Verification items for this drawing (mm, ordinates from the low corner). A direction names the side the tool comes from. Give positions to 0.01 mm unless a question says otherwise; leave off trailing zeros. Loops run counter-clockwise (first coordinate to the right, second up) from the corner with the lowest first, then second, coordinate; pieces in that order, holes last. Notation, with made-up numbers: (43, 27.25) -> (52, 27.25) arc R17 cw to (52, 44.25) -> close; hole circle Ø2 at (55, 51.5). An arc over 180 degrees is marked (long way). Answer in a Markdown table with one row per item. Add a question column.
Q1. Material ranges on probe 1 along Y at (x, z) = (5, 6); probe 2 along Y at (x, z) = (17, 8.5); probe 3 along Y at (x, z) = (16, 2.5), recorded low to high.
Q2. Section check C-C on y = 16. Enter the section's corners in (x, z).
Q3. Section check D-D on y = 7. Enter the section's corners in (x, z).
Q4. Release check for a two-part mould opening along Y. For the marked faces 1, 2, 3 and 4 record: pulls with the +Y half, pulls with the -Y half, needs draft (parallel to the pull), parting line crosses it, or undercut.
Q5. Section check A-A on x = 5. Enter the section's corners in (y, z), and give its area (3 significant figures).
Q6. Section check B-B on z = 5.75. Enter the section's corners in (x, y), and give its area (3 significant figures).
Q7. Set-up check for the marked faces 5 and 6: record each of +Z, -Z, +X, -X, +Y, -Y from which the full face is reachable in a straight line by a thin tool's end or side.
Q8. Gauge pin test, flat ends, axial feed: P1, Ø5, axis at x = 16, y = 16, coming from the +Z side; P2, Ø12, axis at x = 11, y = 7, coming from the +Z side; P3, Ø6.5, axis at x = 2.5, z = 2.5, coming from the +Y side; P4, Ø4, axis at y = 15.5, z = 7, coming from the -X side. Record the tip position at first contact, or that the pin passes through.
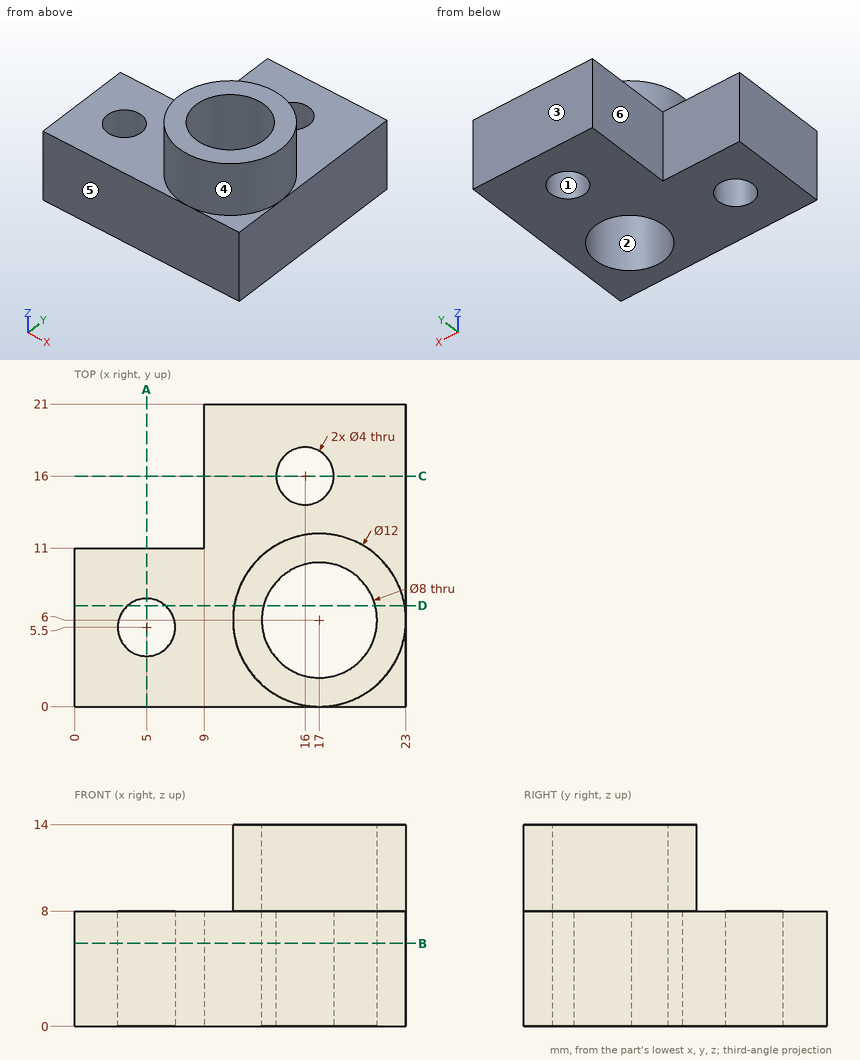
Taken from the geometry:
| question | item | result |
|---|---|---|
| 1 | probe 1 | y = 0 to 3.5, 7.5 to 11 |
| 1 | probe 2 | y = 0 to 2, 10 to 12 |
| 1 | probe 3 | y = 0 to 2.13, 9.87 to 14, 18 to 21 |
| 2 | outline | (9, 0) -> (14, 0) -> (14, 8) -> (9, 8) -> close; (18, 0) -> (23, 0) -> (23, 8) -> (18, 8) -> close |
| 3 | outline | (0, 0) -> (3.68, 0) -> (3.68, 8) -> (0, 8) -> close; (6.32, 0) -> (13.13, 0) -> (13.13, 14) -> (11.08, 14) -> (11.08, 8) -> (6.32, 8) -> close; (20.87, 0) -> (23, 0) -> (23, 8) -> (22.92, 8) -> (22.92, 14) -> (20.87, 14) -> close |
| 4 | face 1 | undercut |
| 4 | face 2 | undercut |
| 4 | face 3 | pulls with the +Y half |
| 4 | face 4 | parting line crosses it |
| 5 | outline | (0, 0) -> (3.5, 0) -> (3.5, 8) -> (0, 8) -> close; (7.5, 0) -> (11, 0) -> (11, 8) -> (7.5, 8) -> close |
| 5 | area | 56.0 mm² |
| 6 | outline | (0, 0) -> (23, 0) -> (23, 21) -> (9, 21) -> (9, 11) -> (0, 11) -> close; hole circle Ø4 at (5, 5.5); hole circle Ø8 at (17, 6); hole circle Ø4 at (16, 16) |
| 6 | area | 318 mm² |
| 7 | face 5 | +Z, -Z, +X, -X, -Y |
| 7 | face 6 | +Z, -Z, -X, +Y |
| 8 | P1 | stops at z = 8 |
| 8 | P2 | stops at z = 14 |
| 8 | P3 | stops at y = 11 |
| 8 | P4 | stops at x = 9 |
